Geometry: final body of the model. Coordinates: model frame, mm. Face numbers are marked on the shaded views. A direction names the side the tool comes from. Coordinates: 2 decimals unless noted, no trailing zeros. Order: outer loops, then holes, each group sorted by start corner. A loop starts at its lowest first (then second) coordinate and runs counter-clockwise, first axis right, second up. Notation, with made-up numbers: M 44,-22 L 97,-22 A9 cw 97,-12 Z; hole C 80,-15 d10. An arc over 180 degrees is marked long. Use CSV: the item, a comma, the result in double quotes. Start each with the question number.
1. Material intervals for line 1 (X direction, y = -40.5, z = 3.5); line 2 (Y direction, x = -18.5, z = -1); line 3 (Y direction, x = -18.75, z = 5.75), sorted ascending.
2. Section query A-A on x = -19.5. Return the cut outline in (y, z), and give its area (3 significant figures).
3. First-contact query: P1, Ø6, axis at x = -15.5, y = -9, coming from the -Z side; P2, Ø7.5, axis at x = -15.32, z = 3.43, coming from the -Y side; P3, Ø6, axis at y = -27, z = -1, coming from the +X side. Flat tips, straight axial feed; report the tip coordinate or a pass-through.
4. Pull-direction query (X, two-part tool) for the marked faces 1, 2, 3 and 4; classes: pulls with the +X half, pulls with the -X half, needs draft (parallel to the pull), parting line crosses it, or undercut.
5. Set-up query: the marked faces 5, 6, 7, 8 and 9. Return all of +Z, -Z, +X, -X, +Y, -Y with unobstructed straight access to the full face (end or side cutting, diameter ignored); none if empty.
6. Section query D-D on y = -11. Return the cut outline in (x, z) (1 decimal), and give its area (3 significant figures).
7. Section query B-B on z = 0.25. Return the cut outline in (x, y), and give its area (3 significant figures).
8. Section query C-C on y = -50. Return the cut outline in (x, z) (1 decimal).
from build123d import *

# Parameters (mm, degrees)
F0_R     = 9.525
F1_DEPTH = 44.45
F2_DEPTH = 19.05
F3_R     = 15.875
F3_R_2   = 9.525
F4_DEPTH = 84.93252
F5_R     = 9.525
F6_DEPTH = 44.45
F8_DEPTH = 25.4
F9_SCALE = 0.5


with BuildPart() as f1:
    # F0 (on Front) → F1 (new body)
    with BuildSketch(Plane.XZ):
        with Locations((-30.6494925171, 6.8525290117)):
            Circle(F0_R)
    extrude(amount=F1_DEPTH)

    # F2 (cut): a face of the model
    f2_faces = [f1.faces().sort_by_distance(p)[0] for p in [
        (-30.6494925171, -44.45, 6.8525290117),
    ]]
    extrude(f2_faces, amount=-F2_DEPTH, mode=Mode.SUBTRACT)

    # F3 (on face) → F4 (join)
    with BuildSketch(Plane.XZ.offset(25.4)):
        with Locations((-30.6494925171, 6.8525290117)):
            Circle(F3_R)
        with Locations((-30.6494925171, 6.8525290117)):
            Circle(F3_R_2, mode=Mode.SUBTRACT)
        with Locations((-30.6494925171, 6.8525290117)):
            Circle(F3_R_2)
    extrude(amount=F4_DEPTH)

    # F5 (on face) → F6 (cut)
    with BuildSketch(Plane.XZ.offset(110.33252)):
        with Locations((-30.6494925171, 6.8525290117)):
            Circle(F5_R)
    extrude(amount=-F6_DEPTH, mode=Mode.SUBTRACT)

    # F7 (on face) → F8 (cut)
    with BuildSketch(Plane.XZ.offset(110.33252)):
        with BuildLine():
            Line((-45.8350943452, 11.4799604934), (-34.2348202137, 22.3173617074))
            ThreePointArc((-34.2348202137, 22.3173617074), (-41.4868937311, 18.4528031432), (-45.8350943452, 11.4799604934))
        make_face()
        with BuildLine():
            Line((-42.2497666486, -3.9848722024), (-45.8350943452, 11.4799604934))
            ThreePointArc((-45.8350943452, 11.4799604934), (-46.1143252129, 3.2672013151), (-42.2497666486, -3.9848722024))
        make_face()
        with BuildLine():
            ThreePointArc((-42.2497666486, -3.9848722024), (-35.2769239989, -8.3330728164), (-27.0641648205, -8.6123036841))
            Line((-27.0641648205, -8.6123036841), (-42.2497666486, -3.9848722024))
        make_face()
        with BuildLine():
            ThreePointArc((-27.0641648205, -8.6123036841), (-19.8120913031, -4.7477451198), (-15.463890689, 2.2250975299))
            Line((-15.463890689, 2.2250975299), (-27.0641648205, -8.6123036841))
        make_face()
        with BuildLine():
            ThreePointArc((-14.7744925171, 6.8525290117), (-15.8817916663, 12.6775300058), (-19.0492183856, 17.6899302257))
            Line((-19.0492183856, 17.6899302257), (-15.463890689, 2.2250975299))
            ThreePointArc((-15.463890689, 2.2250975299), (-14.9477879278, 4.5132774242), (-14.7744925171, 6.8525290117))
        make_face()
        with BuildLine():
            Line((-34.2348202137, 22.3173617074), (-19.0492183856, 17.6899302257))
            ThreePointArc((-19.0492183856, 17.6899302257), (-26.0220610354, 22.0381308398), (-34.2348202137, 22.3173617074))
        make_face()
    extrude(amount=-F8_DEPTH, mode=Mode.SUBTRACT)


with BuildPart() as f1_1:
    # F9: moved
    add(f1.part.scale(F9_SCALE))


solid = f1_1.part
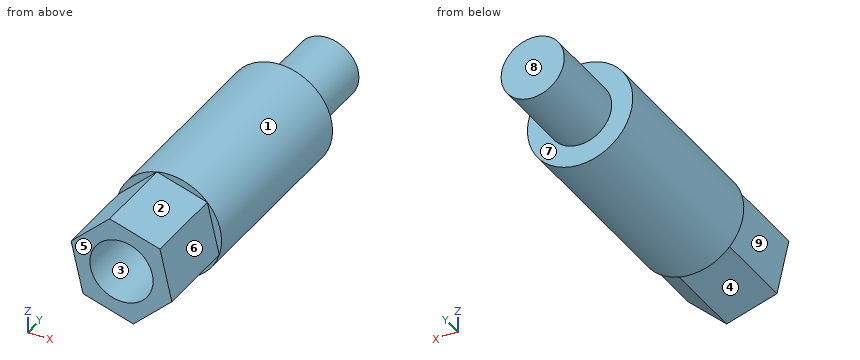
Results list:
1,line 1,"x = -23.26 to -20.09, -10.56 to -7.39"
1,line 2,"y = -55.17 to -12.7"
1,line 3,"y = -32.94 to 0"
2,outline,"M -55.17,-2.49 L -42.47,-2.49 L -42.47,-3.32 L -12.7,-3.32 L -12.7,1.14 L 0,1.14 L 0,5.72 L -12.7,5.72 L -12.7,10.18 L -42.47,10.18 L -42.47,8.93 L -55.17,8.93 L -55.17,5.72 L -32.94,5.72 L -32.94,1.14 L -55.17,1.14 Z"
2,area,"503 mm²"
3,P1,"stops at z = -1.34"
3,P2,"stops at y = -32.94"
3,P3,"stops at x = -7.52"
4,face 1,"parting line crosses it"
4,face 2,"pulls with the +X half"
4,face 3,"undercut"
4,face 4,"pulls with the -X half"
5,face 5,"+Z, -Z, +X, -X, -Y"
5,face 6,"+Z, +X, -Y"
5,face 7,"+Y"
5,face 8,"+Z, -Z, +X, -X, +Y"
5,face 9,"-Z, -X, -Y"
6,outline,"C -15.3,3.4 d9.5"
6,area,"71.3 mm²"
7,outline,"M -22.6,-42.47 L -21.64,-42.47 L -21.64,-55.17 L -18.87,-55.17 L -18.87,-32.94 L -11.78,-32.94 L -11.78,-55.17 L -8.66,-55.17 L -8.66,-42.47 L -8.05,-42.47 L -8.05,-12.7 L -11.78,-12.7 L -11.78,0 L -18.87,0 L -18.87,-12.7 L -22.6,-12.7 Z"
7,area,"530 mm²"
8,outline,"M -22.9,5.7 L -21.1,-2 L -13.5,-4.3 L -7.7,1.1 L -9.5,8.8 L -17.1,11.2 Z; hole C -15.3,3.4 d9.5"
